Check sheet for the drawn part. Datum: minimum x, y, z corner. Units: mm. A direction names the side the tool comes from. Give positions to 0.01 mm unless a question says otherwise; leave off trailing zeros. Order: outer loops, then holes, each group sorted by start corner. A loop starts at its lowest first (then second) coordinate and runs counter-clockwise, first axis right, second up. Notation, with made-up numbers: (73, 78.5) -> (103, 78.5) arc R29 ccw to (103, 111.5) -> close; hole circle Ø2 at (-9, 76.5). An arc over 180 degrees is marked (long way). Return JSON: item names as keys, results as strings. Group by question number.
(1) Cross-section at A-A on z = 9. Enter the section's corners in (x, y) (1 decimal).
(2) Thickness scan on line 1 along X through (y, z) = (7.25, 2.5) (1 decimal); line 2 along Z through (x, y) = (10.5, 10.5); line 3 along Y through (x, z) = (8.75, 8.25) (1 decimal). Record the ranges inside material, lowest first.
(3) Tool access check on the marked faces 1 and 2. Record the directions out of +Z, -Z, +X, -X, +Y, -Y that give a thin tool (end or side, any length) a straight path to the whole face; none if there is none.
(4) Depth check by flat-ended pin: pin 1 Ø6 at (y, z) = (6, 14) entering from -X; pin 2 Ø2 at (y, z) = (10.5, 4.5) entering from -X; pin 3 Ø6 at (x, z) = (4, 9) entering from -Y. Enter the tip coordinate at first touch or a pass-through.
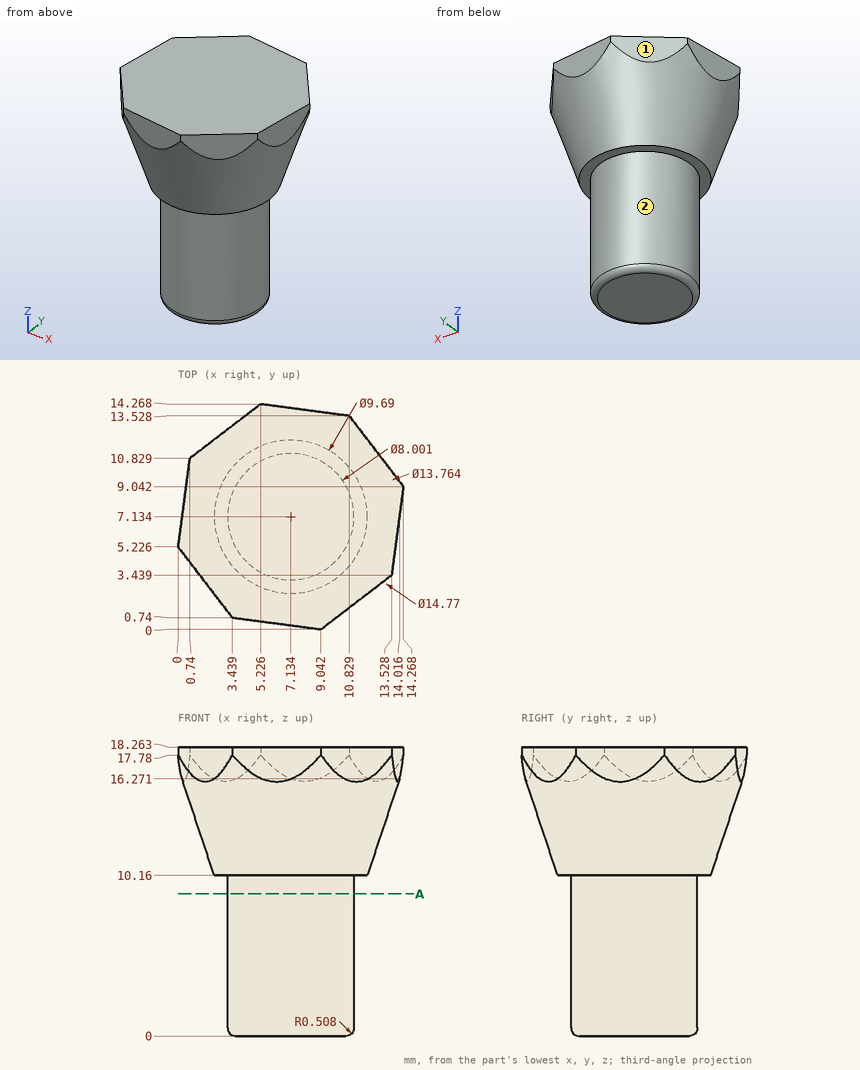
Verdict:
{
 "1": {"outline": "circle Ø8 at (7.1, 7.1)"},
 "2": {"line 1": "3.1 to 11.1", "line 2": "10.16 to 18.26", "line 3": "3.5 to 10.8"},
 "3": {"face 1": "+Z, -Z, -X, +Y", "face 2": "-Z"},
 "4": {"pin 1": "x = 0.1", "pin 2": "x = 3.91", "pin 3": "y = 2.05"}
}
